from build123d import *

# Parameters (mm, degrees)
SKETCH1_W           = 10
SKETCH1_H           = 40
BOSS_EXTRUDE1_DEPTH = 6
SKETCH2_R           = 3.05
CUT_EXTRUDE1_DEPTH  = 3.1
CHAMFER1_SIZE       = 0.25
BOSS_EXTRUDE2_DEPTH = 5
FILLET1_R           = 1.5
FILLET2_R           = 3.5
FILLET3_R           = 1
FILLET4_R           = 1


with BuildPart() as part:
    # Sketch1 → Boss-Extrude1 (new body)
    with BuildSketch(Plane(origin=(0, 0, 0), x_dir=(1, 0, 0), z_dir=(0, 1, 0))):
        with Locations((5, -20)):
            Rectangle(SKETCH1_W, SKETCH1_H)
    extrude(amount=BOSS_EXTRUDE1_DEPTH)

    # Sketch2 → Cut-Extrude1 (cut)
    with BuildSketch(Plane(origin=(0, 6, 0), x_dir=(1, 0, 0), z_dir=(0, 1, 0))):
        with Locations((5, -6)):
            Circle(SKETCH2_R)
    extrude(amount=-CUT_EXTRUDE1_DEPTH, mode=Mode.SUBTRACT)

    # Chamfer1
    chamfer1_edges = [part.edges().sort_by_distance(p)[0] for p in [
        (1.95, 6, 6),
    ]]
    chamfer(chamfer1_edges, length=CHAMFER1_SIZE)

    # Sketch4 → Boss-Extrude2 (add, symmetric)
    with BuildSketch(Plane.ZY.offset(-5)):
        Polygon((12, 6), (12, 13), (40, 13), (40, 11), (39.382855568, 7.5), (37.382855568, 7.5), (36.765711135, 11), (14, 11), (14, 6), align=None)
    extrude(amount=BOSS_EXTRUDE2_DEPTH, both=True)

    # Fillet1
    fillet1_edges = [part.edges().sort_by_distance(p)[0] for p in [
        (5, 11, 14),
    ]]
    fillet(fillet1_edges, radius=FILLET1_R)

    # Fillet2
    fillet2_edges = [part.edges().sort_by_distance(p)[0] for p in [
        (5, 13, 12),
    ]]
    fillet(fillet2_edges, radius=FILLET2_R)

    # Fillet3
    fillet3_edges = [part.edges().sort_by_distance(p)[0] for p in [
        (5, 6, 14),
    ]]
    fillet(fillet3_edges, radius=FILLET3_R)

    # Fillet4
    fillet4_edges = [part.edges().sort_by_distance(p)[0] for p in [
        (5, 11, 36.765711135),
        (5, 7.5, 37.382855568),
        (5, 7.5, 39.382855568),
        (5, 13, 40),
    ]]
    fillet(fillet4_edges, radius=FILLET4_R)


solid = part.part
The listing builds one solid part. Answer for the finished solid, in the listing's coordinates (mm). A direction names the side the tool comes from. Round coordinates to 2 decimals unless told otherwise and drop trailing zeros. Order: outer loops, then holes, each group sorted by start corner. A loop starts at its lowest first (then second) coordinate and runs counter-clockwise, first axis right, second up. Notation, with made-up numbers: M 70,66 L 114,66 A20 cw 114,87 Z; hole C 60.5,-36.75 d11. An arc over 180 degrees is marked long. Answer in a Markdown table with one row per item. Add a question column.
1) The part is cut by section D-D on x = 1.25. Determine the outline of the cut face in (y, z), plus the area to 3 significant figures.
2) The part is cut by section C-C on x = 5. Determine the outline of the cut face in (y, z).
3) Determine the mould class of faces 1 (the face through (5, 8, 12)), 2 (the face through (5.07, 7.74, 37.57)), 3 (the face through (3, 6, 3)) for opening direction Z: pulls with the +Z half, pulls with the -Z half, needs draft (parallel to the pull), parting line crosses it, or undercut.
4) Consider line 1 along X through (y, z) = (3.95, 6); line 2 along Y through (x, z) = (4, 17.5); line 3 along Z through (x, y) = (5, 4.75). Determine where each line is inside the solid, lowest interval first. Write a range as from..to.
5) Flat-ended cylindrical pins translate along their axes: pin 1 Ø2 at (x, y) = (2, 9) entering from -Z; pin 2 Ø0.8 at (x, y) = (3, 8.5) entering from +Z. Find the tip coordinate at first contact, or state that the pin passes through.
6) The part is cut by section B-B on z = 6. Determine the outline of the cut face in (x, y), plus the area to 3 significant figures.
7) The part is cut by section A-A on y = 5. Determine the outline of the cut face in (x, z), plus the area to 3 significant figures.
8) Which of the six approach directions +Z, -Z, +X, -X, +Y, -Y give full straight-line access (tool end or side, diameter ignored) to faces 4 (the face through (5, 11, 26)), 5 (the face through (5, 2.9, 6)), 6 (the face through (4.93, 9.682, 39.768)), 7 (the face through (5.07, 12.715, 39.699)), 8 (the face through (4.9, 11.5, 40))?
Findings below:
| question | item | result |
|---|---|---|
| 1 | outline | M 0,0 L 6,0 L 6,12 L 9.5,12 A3.5 ccw 13,15.5 L 13,39 A1 ccw 12,40 L 11,40 L 8.33,39.53 A1 ccw 7.5,38.54 L 7.5,38.22 A1 ccw 8.33,37.24 L 10.17,36.91 A1 cw 11,35.93 L 11,15.5 A1.5 cw 9.5,14 L 7,14 A1 cw 6,15 L 6,40 L 0,40 Z |
| 1 | area | 313 mm² |
| 2 | outline | M 0,0 L 6,0 L 6,2.7 L 5.75,2.95 L 2.9,2.95 L 2.9,9.05 L 5.75,9.05 L 6,9.3 L 6,12 L 9.5,12 A3.5 ccw 13,15.5 L 13,39 A1 ccw 12,40 L 11,40 L 8.33,39.53 A1 ccw 7.5,38.54 L 7.5,38.22 A1 ccw 8.33,37.24 L 10.17,36.91 A1 cw 11,35.93 L 11,15.5 A1.5 cw 9.5,14 L 7,14 A1 cw 6,15 L 6,40 L 0,40 Z |
| 3 | face 1 | pulls with the -Z half |
| 3 | face 2 | undercut |
| 3 | face 3 | needs draft |
| 4 | line 1 | x = 0..1.95, 8.05..10 |
| 4 | line 2 | y = 0..6, 11..13 |
| 4 | line 3 | z = 0..2.95, 9.05..40 |
| 5 | pin 1 | stops at z = 12 |
| 5 | pin 2 | stops at z = 39.63 |
| 6 | outline | M 0,0 L 10,0 L 10,6 L 8.3,6 L 8.05,5.75 L 8.05,2.9 L 1.95,2.9 L 1.95,5.75 L 1.7,6 L 0,6 Z |
| 6 | area | 41.0 mm² |
| 7 | outline | M 0,0 L 10,0 L 10,40 L 0,40 Z; hole C 5,6 d6.1 |
| 7 | area | 371 mm² |
| 8 | face 4 | +X, -X |
| 8 | face 5 | +Y |
| 8 | face 6 | +Z, +X, -X |
| 8 | face 7 | +Z, +X, -X, +Y |
| 8 | face 8 | +Z, +X, -X, +Y, -Y |
